Check sheet for the modelled part. Datum: model origin and axes. Units: mm. Give positions to 0.01 mm unless a question says otherwise; leave off trailing zeros. Order: outer loops, then holes, each group sorted by start corner. A loop starts at its lowest first (then second) coordinate and runs counter-clockwise, first axis right, second up.
Item 1: Release check for a two-part mould opening along Y. For faces 1 (the flat face through (-15, -2, 0)), 2 (the flat face through (2.7, -14.8, 0)), 3 (the cylindrical face through (-0.29, 14.73, 0.02)), 4 (the flat face through (0, 27.5, 0)) record: released by +Y, released by -Y, zero draft, split by the parting line, or undercut.
Item 2: Sectioned sample at A-A on z = 0.5. Record the boundary of the cut face in (x, y), and give its area (3 significant figures).
Item 3: Gauge pin test, flat end, axial feed: P1, Ø3.5, axis at x = 0, y = 12.5, coming from the -Z side. Record the tip position at first contact, or that the pin passes through.
Item 4: Sectioned sample at C-C on y = 12.5. Record the boundary of the cut face in (x, z), and give its area (3 significant figures).
Item 5: Sectioned sample at D-D on x = 7. Record the boundary of the cut face in (y, z), and give its area (3 significant figures).
Item 6: Sectioned sample at B-B on x = 0. Record the boundary of the cut face in (y, z).
Item 7: Material ranges on line 1 along Y through (x, z) = (1, -0.4); line 2 along Y through (x, z) = (0, -0.55); line 3 along X through (y, z) = (12, 0.3), recorded low to high.
from build123d import *

# Parameters (mm, degrees)
SKETCH1_W           = 30
SKETCH1_H           = 55
BOSS_EXTRUDE1_DEPTH = 1.5
CHAMFER1_SIZE       = 3
SKETCH2_R           = 2.25
CUT_EXTRUDE1_DEPTH  = 10
CHAMFER2_SIZE       = 25


with BuildPart() as part:
    # Sketch1 → Boss-Extrude1 (new, symmetric)
    with BuildSketch(Plane.XY):
        Rectangle(SKETCH1_W, SKETCH1_H)
    extrude(amount=BOSS_EXTRUDE1_DEPTH, both=True)

    # Chamfer1
    chamfer1_edges = [part.edges().sort_by_distance(p)[0] for p in [
        (-15, 27.5, 0),
        (15, 27.5, 0),
    ]]
    chamfer(chamfer1_edges, length=CHAMFER1_SIZE)

    # Sketch2 → Cut-Extrude1 (cut)
    with BuildSketch(Plane.XY.offset(1.5)):
        with Locations((0, 12.5)):
            Circle(SKETCH2_R)
    extrude(amount=-CUT_EXTRUDE1_DEPTH, mode=Mode.SUBTRACT)

    # Chamfer2
    chamfer2_edges = [part.edges().sort_by_distance(p)[0] for p in [
        (15, -27.5, 0),
    ]]
    chamfer(chamfer2_edges, length=CHAMFER2_SIZE)


solid = part.part
Report:
1. face 1: zero draft
1. face 2: released by -Y
1. face 3: undercut
1. face 4: released by +Y
2. outline: (-15, -27.5) - (-10, -27.5) - (15, -2.5) - (15, 24.5) - (12, 27.5) - (-12, 27.5) - (-15, 24.5) - close; hole circle Ø4.5 at (0, 12.5)
2. area: 1,310 mm2
3. P1: passes through
4. outline: (-15, -1.5) - (-2.25, -1.5) - (-2.25, 1.5) - (-15, 1.5) - close; (2.25, -1.5) - (15, -1.5) - (15, 1.5) - (2.25, 1.5) - close
4. area: 76.5 mm2
5. outline: (-10.5, -1.5) - (27.5, -1.5) - (27.5, 1.5) - (-10.5, 1.5) - close
5. area: 114 mm2
6. outline: (-17.5, -1.5) - (10.25, -1.5) - (10.25, 1.5) - (-17.5, 1.5) - close; (14.75, -1.5) - (27.5, -1.5) - (27.5, 1.5) - (14.75, 1.5) - close
7. line 1: y = -16.5 to 10.48, 14.52 to 27.5
7. line 2: y = -17.5 to 10.25, 14.75 to 27.5
7. line 3: x = -15 to -2.19, 2.19 to 15
